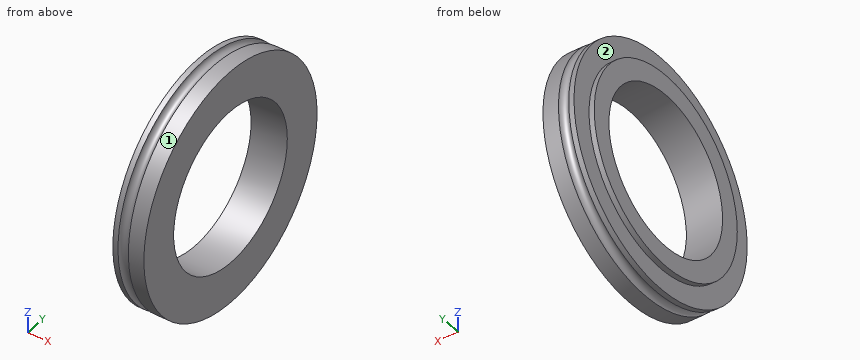
```python
from build123d import *

# Parameters (mm, degrees)
F0_R     = 11.5
F1_DEPTH = 3
F2_R     = 9.5
F3_DEPTH = 0.5
F5_D     = 15.1
F5_DEPTH = 30
F5_TIP   = 4.5364976737
F6_R     = 0.5


with BuildPart() as f1:
    # F0 (on Right) → F1 (new body)
    with BuildSketch(Plane.YZ):
        Circle(F0_R)
    extrude(amount=F1_DEPTH)

    # F2 (on face) → F3 (join)
    with BuildSketch(Plane(origin=(0, 0, 0), x_dir=(0, -1, 0), z_dir=(-1, 0, 0))):
        Circle(F2_R)
    extrude(amount=F3_DEPTH)

    # F5
    with Locations(Plane(origin=(-0.5, 0, 0), x_dir=(0, -1, 0), z_dir=(-1, 0, 0))):
        with Locations((0, 0)):
            Hole(F5_D / 2, depth=F5_DEPTH)
            with Locations((0, 0, -(F5_DEPTH + F5_TIP / 2))):  # 118° drill point
                Cone(0, F5_D / 2, F5_TIP, mode=Mode.SUBTRACT)

    # F7: sweep along a path in F7_path
    with BuildLine(Plane(origin=(0, 11.5, 0), x_dir=(0, 0, 1), z_dir=(1, 0, 0))) as f7_path:
        CenterArc((0, 11.5), 11.5, 0, 360)
    # F6 (on Front) → F7 (sweep, cut)
    with BuildSketch(Plane.XZ):
        with Locations((1, -11.5)):
            Circle(F6_R)
    sweep(path=f7_path.line, mode=Mode.SUBTRACT)


solid = f1.part
```
Source: CAD feature listing. Evaluate the final solid. Frame: model axes, mm. Face numbers are marked on the shaded views. A direction names the side the tool comes from. Round coordinates to 2 decimals unless told otherwise and drop trailing zeros. Write each loop counter-clockwise with the first axis right and the second up, starting at its lowest first coordinate (ties: lowest second). Pieces come first, ordered by that corner, then holes. Notation, with made-up numbers: M -40,35.25 L -24,35.25 A33 ccw -24,66.25 Z; hole C 83,18 d11. An arc over 180 degrees is marked long. Answer as a JSON object with one key per item and string values. Group by question number.
(1) Ray query, line 1 (Z direction, x = 1.95, y = 0); line 2 (X direction, y = 8, z = -8); line 3 (Y direction, x = 2.35, z = -5.25). Return the intervals inside material, ascending. Write a range as [from, to].
(2) First-contact query: pin 1 (1 mm diameter, centred on x = 0.5, z = -6.5, fed in from +Y). Flat tip, straight axial feed; report the tip coordinate or a pass-through.
(3) Section query A-A on y = 0. Output: boundary loops of the cut face in (x, z).
(4) Reachability of the marked faces 1 and 2 from +Z, -Z, +X, -X, +Y, -Y: full face, straight path, thin tool, end or side. Return the list, or none.
(5) Section query C-C on x = 1.95. Output: boundary loops of the cut face in (y, z), then the cut area to 3 significant figures.
Computed values:
{
 "1": {"line 1": "[-11.5, -7.55], [7.55, 11.5]", "line 2": "[0, 0.54], [1.46, 3]", "line 3": "[-10.23, -5.43], [5.43, 10.23]"},
 "2": {"pin 1": "y = 9.81"},
 "3": {"outline": "M -0.5,-9.5 L 0,-9.5 L 0,-11.5 L 0.5,-11.5 A0.5 cw 1.5,-11.5 L 3,-11.5 L 3,-7.55 L -0.5,-7.55 Z; M -0.5,7.55 L 3,7.55 L 3,11.5 L 1.5,11.5 A0.5 cw 0.5,11.5 L 0,11.5 L 0,9.5 L -0.5,9.5 Z"},
 "4": {"face 1": "+X, -X", "face 2": "-X"},
 "5": {"outline": "C 0,0 d23; hole C 0,0 d15.1", "area": "236 mm^2"}
}
